Check sheet for the drawn part. Datum: minimum x, y, z corner. Units: mm. A direction names the side the tool comes from. Coordinates: 2 decimals unless noted, no trailing zeros. Loops run counter-clockwise (first coordinate to the right, second up) from the corner with the lowest first, then second, coordinate; pieces in that order, holes last.
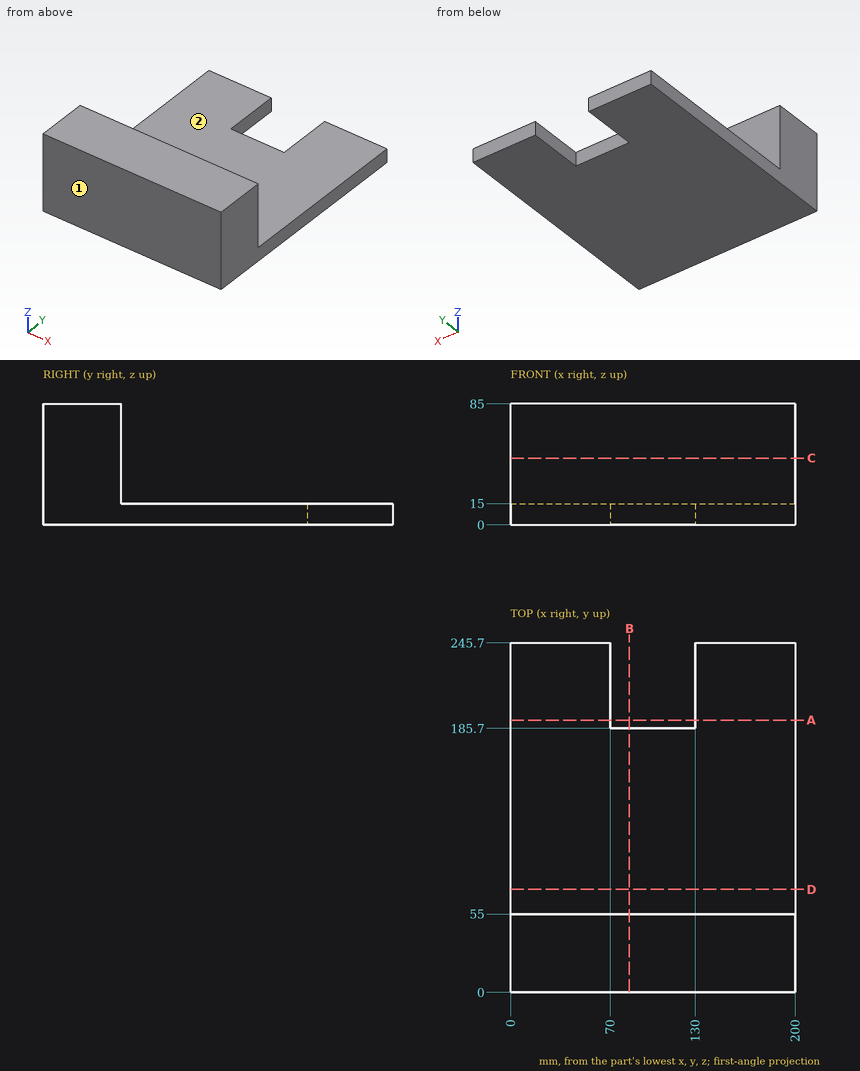
1) Scan lines: line 1 (Z direction, x = 43.5, y = 212); line 2 (Y direction, x = 49, z = 45); line 3 (Y direction, x = 124, z = 4.5). Record each from-to range of solid material in increasing order.
Answer sheet:
line 1: z = 0 to 15
line 2: y = 0 to 55
line 3: y = 0 to 185.7
2) Section check C-C on z = 47. Enter the section's corners in (x, y).
Answer sheet:
outline: (0, 0) - (200, 0) - (200, 55) - (0, 55) - close
3) Section check D-D on y = 72.5. Enter the section's corners in (x, z), plus the area to 3 significant figures.
Answer sheet:
outline: (0, 0) - (200, 0) - (200, 15) - (0, 15) - close
area: 3,000 mm2
4) Set-up check for the marked faces 1 and 2: record each of +Z, -Z, +X, -X, +Y, -Y from which the full face is reachable in a straight line by a thin tool's end or side.
Answer sheet:
face 1: +Z, -Z, +X, -X, -Y
face 2: +Z, +X, -X, +Y
5) Section check A-A on y = 191.5. Enter the section's corners in (x, z).
Answer sheet:
outline: (0, 0) - (70, 0) - (70, 15) - (0, 15) - close; (130, 0) - (200, 0) - (200, 15) - (130, 15) - close
6) Depth check by flat-ended pin: pin 1 (1.5 mm diameter, centred on x = 136, y = 195, fed in from +Z); pin 2 (16.5 mm diameter, centred on x = 95, z = 11, fed in from +Y); pin 3 (8 mm diameter, centred on x = 21, z = 31, fed in from +Y). Enter the tip coordinate at first touch or a pass-through.
Answer sheet:
pin 1: stops at z = 15
pin 2: stops at y = 185.7
pin 3: stops at y = 55
7) Section check B-B on x = 83.5. Enter the section's corners in (y, z).
Answer sheet:
outline: (0, 0) - (185.7, 0) - (185.7, 15) - (55, 15) - (55, 85) - (0, 85) - close
